```python
from build123d import *

# Parameters (mm, degrees)
F1_DEPTH = 5
F0_W     = 5.95
F0_H     = 6.9
F2_DEPTH = 2.5
F5_R     = 0.95
F6_DEPTH = 1.9
F4_R     = 0.95
F7_DEPTH = 1.9


with BuildPart() as f1:
    # F0 (on Front) → F1 (new body)
    with BuildSketch(Plane.XZ):
        Polygon((64.440538, -6.86276), (64.440538, 0.03724), (36.890538, 0.03724), (36.890538, -2.96276), (23.390538, -2.96276), (23.390538, 0.03724), (16.890538, 0.03724), (16.890538, -2.96276), (3.390538, -2.96276), (3.390538, 0.03724), (-3.109462, 0.03724), (-3.109462, -2.96276), (-16.609462, -2.96276), (-16.609462, 0.03724), (-23.109462, 0.03724), (-23.109462, -2.96276), (-36.609462, -2.96276), (-36.609462, 0.03724), (-64.159462, 0.03724), (-64.159462, -6.86276), align=None)
    extrude(amount=F1_DEPTH)

    # F0 (on Front) → F2 (join)
    with BuildSketch(Plane.XZ):
        with Locations((-67.134462, -3.41276)):
            Rectangle(F0_W, F0_H)
        with Locations((67.415538, -3.41276)):
            Rectangle(F0_W, F0_H)
    extrude(amount=F2_DEPTH)

    # F5 (on face) → F6 (join)
    with BuildSketch(Plane.XY.offset(0.03724)):
        with Locations((-50.384462, -2.5)):
            Circle(F5_R)
    extrude(amount=F6_DEPTH)

    # F4 (on face) → F7 (join)
    with BuildSketch(Plane.XY.offset(0.03724)):
        with Locations((50.665538, -2.5)):
            Circle(F4_R)
    extrude(amount=F7_DEPTH)


solid = f1.part
```
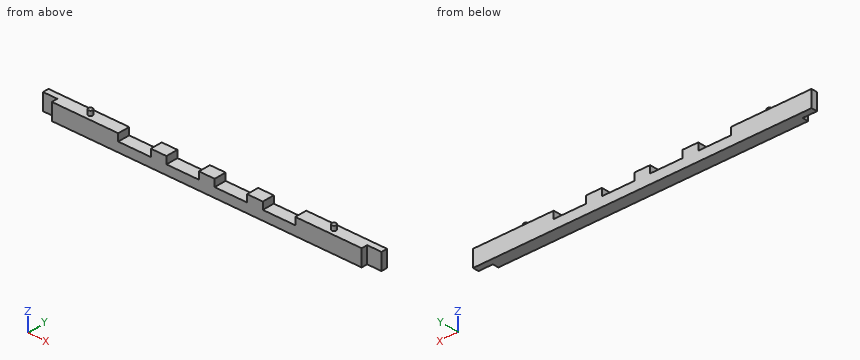
Part model, mm, in its own coordinate system. Round coordinates to 2 decimals unless told otherwise and drop trailing zeros. Loops run counter-clockwise (first coordinate to the right, second up) from the corner with the lowest first, then second, coordinate; pieces in that order, holes last.
Item 1: Cut at A-A, the plane z = -5. Give the cut face in (x, y), then the cut area to 3 significant figures.
Item 2: Drill centre lines: line 1 (X direction, y = -4.7, z = -1.5); line 2 (X direction, y = -2.4, z = -1.75); line 3 (Z direction, x = 54.5, y = -0.35). Where is each one in solid material? Low to high.
Item 3: Cut at C-C, the plane x = -11. Give the cut face in (y, z), then the cut area to 3 significant figures.
Item 4: Drop flat-ended pins along their axis: P1, Ø0.9, axis at y = -3.5, z = -1.5, coming from the -X side; P2, Ø1.5, axis at x = 33, y = -3, coming from the +Z side; P3, Ø3, axis at y = -3.5, z = -5.5, coming from the -X side; P4, Ø3, axis at x = 68, z = -2, coming from the -Y side. Give the stop position or say it passes through.
Item 5: Cut at B-B, the plane x = 54. Give the cut face in (y, z).
A:
1. outline: (-70.11, -2.5) - (-64.16, -2.5) - (-64.16, -5) - (64.44, -5) - (64.44, -2.5) - (70.39, -2.5) - (70.39, 0) - (-70.11, 0) - close
1. area: 673 mm2
2. line 1: x = -64.16 to -36.61, -23.11 to -16.61, -3.11 to 3.39, 16.89 to 23.39, 36.89 to 64.44
2. line 2: x = -70.11 to -36.61, -23.11 to -16.61, -3.11 to 3.39, 16.89 to 23.39, 36.89 to 70.39
2. line 3: z = -6.86 to 0.04
3. outline: (-5, -6.86) - (0, -6.86) - (0, -2.96) - (-5, -2.96) - close
3. area: 19.5 mm2
4. P1: stops at x = -64.16
4. P2: stops at z = -2.96
4. P3: stops at x = -70.11
4. P4: stops at y = -2.5
5. outline: (-5, -6.86) - (0, -6.86) - (0, 0.04) - (-5, 0.04) - close
